Could you check a few things on this model? Use its own coordinates, in mm. Coordinates: 2 decimals unless noted, no trailing zeros. Order: outer loops, then holes, each group sorted by start corner. A loop starts at its lowest first (then second) coordinate and runs counter-clockwise, first axis right, second up. Notation, with made-up numbers: (43, 67.5) -> (90, 67.5) arc R25 ccw to (90, 81.5) -> close; hole circle Ø2 at (80, 85.5). An arc over 180 degrees is marked (long way). Put each result on its own line as item: value. Start each with the question number.
Q1. If we section it at B-B (x = -19.05): Please give me the cut outline in (y, z), and give its area (3 significant figures).
Q2. If we section it at D-D (y = 12): Please give me the cut outline in (x, z).
Q3. If we section it at A-A (z = -5): Please give me the cut outline in (x, y), and give its area (3 significant figures).
Q4. Will these pins go through, and if not, where does the flat tip stop? pin 1 (3 mm diameter, centred on x = 2, z = -3.5, fed in from +Y); pin 2 (5.5 mm diameter, centred on x = -76.2, y = 101.6, fed in from +Z); pin 3 (3 mm diameter, centred on x = -46, z = -5.5, fed in from -Y); pin 4 (4 mm diameter, centred on x = -19.05, y = 31.75, fed in from +Z).
Q5. Please list where these lines run through material, in increasing order: line 1 along Y through (x, z) = (-19.05, -1.25); line 2 along Y through (x, z) = (-6, -5); line 3 along X through (y, z) = (33.5, -5.75).
Q6. If we section it at C-C (y = 101.6): Please give me the cut outline in (x, z), and give its area (3 significant figures).
from build123d import *

# Parameters (mm, degrees)
SKETCH1_R           = 2.286
SKETCH1_R_2         = 2.159
BOSS_EXTRUDE1_DEPTH = 6.35
FILLET1_R           = 6.35


with BuildPart() as part:
    # Sketch1 → Boss-Extrude1 (new body)
    with BuildSketch(Plane.XY):
        with BuildLine():
            Line((0, 0), (-25.4, 0))
            Line((-25.4, 0), (-81.711981324, 98.447134338))
            ThreePointArc((-81.711981324, 98.447134338), (-80.122257521, 106.593835794), (-71.830872801, 106.207952639))
            Line((-71.830872801, 106.207952639), (0, 38.1))
            Line((0, 38.1), (15.393399204, 0))
            Line((15.393399204, 0), (0, 0))
        make_face()
        with Locations((-6.35, 6.35)):
            Circle(SKETCH1_R, mode=Mode.SUBTRACT)
        with Locations((-19.05, 31.75)):
            Circle(SKETCH1_R, mode=Mode.SUBTRACT)
        with Locations((-76.2, 101.6)):
            Circle(SKETCH1_R_2, mode=Mode.SUBTRACT)
    extrude(amount=-BOSS_EXTRUDE1_DEPTH)

    # Fillet1
    fillet1_edges = [part.edges().sort_by_distance(p)[0] for p in [
        (15.393399204, 0, -3.175),
    ]]
    fillet(fillet1_edges, radius=FILLET1_R)


solid = part.part
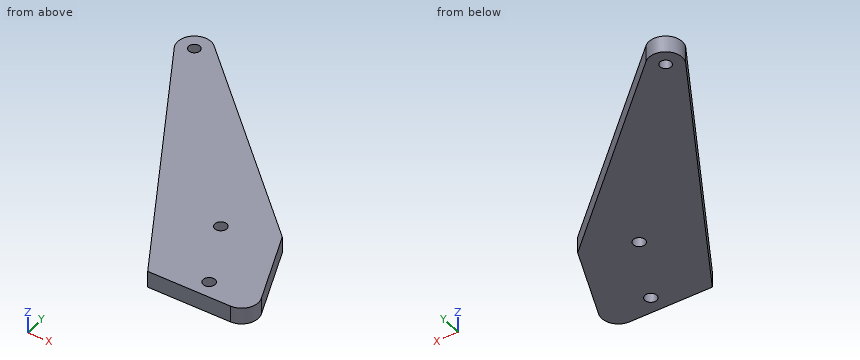
The answers:
1. outline: (0, -6.35) -> (29.46, -6.35) -> (29.46, 0) -> (0, 0) -> close; (34.04, -6.35) -> (56.16, -6.35) -> (56.16, 0) -> (34.04, 0) -> close
1. area: 328 mm^2
2. outline: (-32.26, -6.35) -> (10.55, -6.35) -> (10.55, 0) -> (-32.26, 0) -> close
3. outline: (-81.71, 98.45) -> (-25.4, 0) -> (5.98, 0) arc R6.35 ccw to (11.87, 8.73) -> (0, 38.1) -> (-71.83, 106.21) arc R6.35 ccw to start; hole circle Ø4.32 at (-76.2, 101.6); hole circle Ø4.57 at (-19.05, 31.75); hole circle Ø4.57 at (-6.35, 6.35)
3. area: 3,700 mm^2
4. pin 1: y = 36.86
4. pin 2: z = 0
4. pin 3: y = 33.39
4. pin 4: through
5. line 1: 0 to 29.46, 34.04 to 56.16
5. line 2: 0 to 4.09, 8.61 to 43.79
5. line 3: -44.56 to -20.52, -17.58 to 1.86
6. outline: (-82.55, -6.35) -> (-78.36, -6.35) -> (-78.36, 0) -> (-82.55, 0) -> close; (-74.04, -6.35) -> (-66.97, -6.35) -> (-66.97, 0) -> (-74.04, 0) -> close
6. area: 71.5 mm^2
